Autodesk Inventor part; units mm, degrees
ref_plane "YZ Plane" through (0, 0, 0) normal (1, 0, 0) x (0, 1, 0)
ref_plane "XZ Plane" through (0, 0, 0) normal (0, 1, 0) x (-1, 0, 0)
ref_plane "XY Plane" through (0, 0, 0) normal (0, 0, 1) x (1, 0, 0)
sketch "Sketch1" plane through (0, 0, 0) normal (0, 1, 0) x (-1, 0, 0)
  line L0 (34.697, 0) -> (-17.3485, -30.0485)
  line L1 (-17.3485, -30.0485) -> (-17.3485, 30.0485)
  line L2 (-17.3485, 30.0485) -> (34.697, 0)
  line L3 (12.7, -12.7) -> (-12.7, -12.7) construction
  line L4 (-12.7, -12.7) -> (-12.7, 12.7) construction
  line L5 (-12.7, 12.7) -> (12.7, 12.7) construction
  line L6 (12.7, 12.7) -> (12.7, -12.7) construction
  line L7 (-17.3485, 15) -> (-117.3485, 15)
  line L8 (-117.3485, 15) -> (-117.3485, -15)
  line L9 (-117.3485, -15) -> (-17.3485, -15)
  line L10 (-4.3161, -22.5243) -> (45.6839, -109.1268)
  line L11 (45.6839, -109.1268) -> (71.6646, -94.1268)
  line L12 (71.6646, -94.1268) -> (21.6646, -7.5243)
  line L13 (0, 0) -> (58.6743, -101.6268) construction
  line L14 (0, 0) -> (-117.3485, 0) construction
  line L15 (-4.3161, 22.5243) -> (45.6839, 109.1268)
  line L16 (45.6839, 109.1268) -> (71.6646, 94.1268)
  line L17 (71.6646, 94.1268) -> (21.6646, 7.5243)
  line L18 (58.6743, 101.6268) -> (0, 0) construction
  line L19 (11.5, -11.5) -> (-11.5, -11.5)
  line L20 (-11.5, -11.5) -> (-11.5, 11.5)
  line L21 (-11.5, 11.5) -> (11.5, 11.5)
  line L22 (11.5, 11.5) -> (11.5, -11.5)
  circle A0 centre (-12, 20.7846) radius 2.5
  line L23 (0, 0) -> (-17.3485, 30.0485) construction
  line L24 (0, 0) -> (-17.3485, -30.0485) construction
  line L25 (0, 0) -> (34.697, 0) construction
  circle A1 centre (-12, -20.7846) radius 2.5
  circle A2 centre (24, 0) radius 2.5
  dimension "d1" = 25.4
  dimension "d2" = 30
  dimension "d3" = 100
  dimension "d4" = 30
  dimension "d5" = 100
  dimension "d6" = 120
  dimension "d7" = 30
  dimension "d8" = 100
  dimension "d9" = 120
  dimension "d10" = 23
  dimension "d21" = 5
  dimension "d22" = 24
  dimension "d23" = 5
  dimension "d24" = 5
  dimension "d25" = 24
  dimension "d26" = 24
extrude "Extrusion1" add sketch "Sketch1" against normal blind 30 contours L0 L1 L2 | L12 L11 L10 L0 | L2 L15 L16 L17 | L9 L8 L7 L1 | L19 L20 L21 L22 | A0 | A1 | A2
sketch "Sketch2" plane through (17.3485, 0, 15) normal (0, 0, 1) x (1, 0, 0)
  line L0 (0, 0) -> (100, 0) construction
  line L1 (0, -30) -> (0, 0) construction
  line L2 (100, -30) -> (0, -30) construction
  line L3 (100, 0) -> (100, -30)
  line L4 (0, 0) -> (100, -83.91)
  line L5 (100, 0) -> (100, -30)
  line L6 (100, -83.91) -> (100, 0)
  line L7 (0, 0) -> (100, 0)
  point P0 (-17.3485, 0)
  dimension "d13" = 40
extrude "Extrusion2" cut sketch "Sketch2" against normal up to next
pattern_circular "Circular Pattern1" count 3 over 360 about axis through (0, -10, 0) along (0, 1, 0) of "Extrusion2"
extrude "Extrusion3" add sketch "Sketch1" along normal blind 25.4 contours L19 L20 L21 L22
extrude "Extrusion4" cut sketch "Sketch1" against normal up to next contours A0 | A1 | A2
equation "\"d4\" = d2"
equation "\"d5\" = d3"
equation "\"d7\" = d2"
equation "\"d8\" = d3"
equation "\"d9\" = d6"
equation "\"d23\" = d21"
equation "\"d24\" = d21"
properties part number "core"
Part model, mm, in its own coordinate system. A direction names the side the tool comes from. Coordinates: 2 decimals unless noted, no trailing zeros. Write each loop counter-clockwise with the first axis right and the second up, starting at its lowest first coordinate (ties: lowest second). Pieces come first, ordered by that corner, then holes. Notation, with made-up numbers: (24.25, 19.5) - (40.25, 19.5) arc R19 ccw to (40.25, 56.5) - close; hole circle Ø3 at (69, -14.75). An arc over 180 degrees is marked (long way). Put each result on its own line as item: value.
1. Band-saw the part on B-B (z = -26.5). Write the cut outline in (x, y), then the cut area to 3 significant figures.
Final values:
outline: (-32.62, -30) - (2.02, -30) - (2.02, -3.85) - (-32.62, -18.39) - close; (11.2, -30) - (17.35, -30) - (17.35, 0) - (11.2, 0) - close
area: 838 mm²
2. Band-saw the part on D-D (y = -2.5). Write the cut outline in (x, z).
Final values:
outline: (-34.7, 0) - (-21.66, -7.52) - (-23.15, -10.1) - (2.83, -25.1) - (4.32, -22.52) - (17.35, -30.05) - (17.35, -15) - (20.33, -15) - (20.33, 15) - (17.35, 15) - (17.35, 30.05) - (4.32, 22.52) - (2.83, 25.1) - (-23.15, 10.1) - (-21.66, 7.52) - close; hole circle Ø5 at (-24, 0); hole circle Ø5 at (12, -20.78); hole circle Ø5 at (12, 20.78)
3. Flat gauge pins, fed straight in: pin 1 Ø3 at (x, z) = (12, -20.78) entering from -Y; pin 2 Ø4.5 at (y, z) = (-8, -21.5) entering from +X; pin 3 Ø6 at (x, z) = (-28.5, 40.5) entering from +Y; pin 4 Ø6.5 at (x, z) = (12, 20.78) entering from -Y. Where does each tip first touch, or does it go through?
Final values:
pin 1: passes through
pin 2: stops at x = 17.35
pin 3: stops at y = -24.31
pin 4: stops at y = -30
4. Band-saw the part on C-C (y = 11). Write the cut outline in (x, z).
Final values:
outline: (-11.5, -11.5) - (11.5, -11.5) - (11.5, 11.5) - (-11.5, 11.5) - close
5. Probe line 1 along Z through (x, y) = (12, -14.5); line 2 along Z through (x, y) = (-30, -15); line 3 along Z through (x, y) = (-22.5, -5.5). List the from-to ranges inside material, lowest first. Write a range as [from, to].
Final values:
line 1: z = [-26.96, -23.28], [-18.28, 18.28], [23.28, 26.96]
line 2: z = [-23.35, -21.96], [-2.71, 2.71], [21.96, 23.35]
line 3: z = [-14.61, -8.97], [-7.04, -2], [2, 7.04], [8.97, 14.61]
6. 3-axis set-ups, long thin cutter, end or side, ignore diameter. For faces 1 (the flat face through (-0.524, -21.457, -30.908)), 2 (the flat face through (0, 13, 11.5)), 3 (the flat face through (-28.09, -14.79, 3.815)), 4 (the flat face through (28, -21, -15)), 5 (the flat face through (0, 13, -11.5)): which of +Z, -Z, +X, -X, +Y, -Y reach the whole face in a straight line?
Final values:
face 1: -Z, +Y, -Y
face 2: +Z, +X, -X, +Y
face 3: -X, +Y, -Y
face 4: -Z, +X, +Y, -Y
face 5: -Z, +X, -X, +Y
7. Band-saw the part on A-A (x = -24). Write the cut outline in (y, z).
Final values:
outline: (-30, -47.46) - (-3.92, -11.57) - (-30, -11.57) - close; (-30, -6.18) - (0, -6.18) - (0, -2.5) - (-30, -2.5) - close; (-30, 2.5) - (0, 2.5) - (0, 6.18) - (-30, 6.18) - close; (-30, 11.57) - (-3.92, 11.57) - (-30, 47.46) - close
8. Two-plate mould, pull along Z, no slides. Class faces 6 (the flat face through (13, 0, -2)), 7 (the flat face through (-17.67, -14.79, 30.18)), 8 (the flat face through (-26.755, -21.457, 16.342)): +Z half, -Z half, draft (parallel to the pull), parting line (faces both ways), or undercut.
Final values:
face 6: draft
face 7: +Z half
face 8: undercut
